```python
from build123d import *

# Parameters (mm, degrees)
SKETCH1_R           = 2.5
BOSS_EXTRUDE1_DEPTH = 2.54


with BuildPart() as part:
    # Sketch1 → Boss-Extrude1 (new body)
    with BuildSketch(Plane(origin=(0, 0, 0), x_dir=(1, 0, 0), z_dir=(0, 1, 0))):
        with BuildLine():
            Line((-127, 38.1), (-127, 23.495))
            ThreePointArc((-127, 23.495), (-124.768153673, 18.106846327), (-119.38, 15.875))
            Line((-119.38, 15.875), (119.38, 15.875))
            ThreePointArc((119.38, 15.875), (124.768153673, 18.106846327), (127, 23.495))
            Line((127, 23.495), (127, 38.1))
            Line((127, 38.1), (146.05, 38.1))
            Line((146.05, 38.1), (146.05, -38.1))
            Line((146.05, -38.1), (127, -38.1))
            Line((127, -38.1), (127, -15.875))
            Line((127, -15.875), (-127, -15.875))
            Line((-127, -15.875), (-127, -38.1))
            Line((-127, -38.1), (-146.05, -38.1))
            Line((-146.05, -38.1), (-146.05, 38.1))
            Line((-146.05, 38.1), (-127, 38.1))
        make_face()
        with Locations(Location((136.525, 20.32, 0), (0, 0, 270))):
            Circle(SKETCH1_R, mode=Mode.SUBTRACT)
        with Locations(Location((136.525, -20.32, 0), (0, 0, 270))):
            Circle(SKETCH1_R, mode=Mode.SUBTRACT)
        with Locations(Location((-136.525, 20.32, 0), (0, 0, 90))):
            Circle(SKETCH1_R, mode=Mode.SUBTRACT)
        with Locations(Location((-136.525, -20.32, 0), (0, 0, 90))):
            Circle(SKETCH1_R, mode=Mode.SUBTRACT)
    extrude(amount=BOSS_EXTRUDE1_DEPTH)


solid = part.part
```
Check sheet for the modelled part. Datum: model origin and axes. Units: mm. A direction names the side the tool comes from. Give positions to 0.01 mm unless a question says otherwise; leave off trailing zeros. Order: outer loops, then holes, each group sorted by start corner. A loop starts at its lowest first (then second) coordinate and runs counter-clockwise, first axis right, second up. Notation, with made-up numbers: M 62,2.5 L 92,2.5 A37 ccw 92,39.5 Z; hole C 72,31 d2. An arc over 180 degrees is marked long. Answer in a Markdown table with one row per item. Add a question column.
Q1. Sectioned sample at D-D, the plane x = 10. Record the boundary of the cut face in (y, z) (3 decimals).
Q2. Access from +Z, -Z, +X, -X, +Y, -Y to the whole of each face (thin tool, end or side, straight path). Record for faces 1 (the cylindrical face through (-124.83, 1.25, -18.17)), 2 (the flat face through (2, 0, -1)).
Q3. Sectioned sample at A-A, the plane z = 20.32. Record the boundary of the cut face in (x, y) (3 decimals).
Q4. Release check for a two-part mould opening along Z. For faces 3 (the flat face through (2, 2.54, -1)), 4 (the cylindrical face through (-139.004, 1.252, -19.995)), 5 (the cylindrical face through (124.71, 1.25, -18.05)) record: released by +Z, released by -Z, zero draft, split by the parting line, or undercut.
Q5. Sectioned sample at B-B, the plane y = 1.5. Record the boundary of the cut face in (x, z) (3 decimals), and give its area (3 significant figures).
Q6. Sectioned sample at C-C, the plane z = -20.32. Record the boundary of the cut face in (x, y) (3 decimals).
Q7. Gauge pin test, flat end, axial feed: pin 1 Ø4 at (x, z) = (136.525, -20.32) entering from +Y. Record the tip position at first contact, or that the pin passes through.
Q8. Thickness scan on L1, parallel to X at y = 1.3, z = 20.32 (3 decimals); L2, parallel to X at y = 1.65, z = -20.32 (3 decimals); L3, parallel to X at y = 0.6, z = 34.5. Record the ranges inside material, lowest first.
Verdict:
| question | item | result |
|---|---|---|
| 1 | outline | M 0,-15.875 L 2.54,-15.875 L 2.54,15.875 L 0,15.875 Z |
| 2 | face 1 | -Z, +Y, -Y |
| 2 | face 2 | +Z, -Z, +X, -X, -Y |
| 3 | outline | M -146.05,0 L -139.025,0 L -139.025,2.54 L -146.05,2.54 Z; M -134.025,0 L -127,0 L -127,2.54 L -134.025,2.54 Z; M 127,0 L 134.025,0 L 134.025,2.54 L 127,2.54 Z; M 139.025,0 L 146.05,0 L 146.05,2.54 L 139.025,2.54 Z |
| 4 | face 3 | zero draft |
| 4 | face 4 | undercut |
| 4 | face 5 | released by -Z |
| 5 | outline | M -146.05,-38.1 L -127,-38.1 L -127,-23.495 A7.62 cw -119.38,-15.875 L 119.38,-15.875 A7.62 cw 127,-23.495 L 127,-38.1 L 146.05,-38.1 L 146.05,38.1 L 127,38.1 L 127,15.875 L -127,15.875 L -127,38.1 L -146.05,38.1 Z; hole C -136.525,-20.32 d5; hole C -136.525,20.32 d5; hole C 136.525,-20.32 d5; hole C 136.525,20.32 d5 |
| 5 | area | 10,900 mm² |
| 6 | outline | M -146.05,0 L -139.025,0 L -139.025,2.54 L -146.05,2.54 Z; M -134.025,0 L -126.307,0 L -126.307,2.54 L -134.025,2.54 Z; M 126.307,0 L 134.025,0 L 134.025,2.54 L 126.307,2.54 Z; M 139.025,0 L 146.05,0 L 146.05,2.54 L 139.025,2.54 Z |
| 7 | pin 1 | through |
| 8 | L1 | -146.05 to -139.025, -134.025 to -127, 127 to 134.025, 139.025 to 146.05 |
| 8 | L2 | -146.05 to -139.025, -134.025 to -126.307, 126.307 to 134.025, 139.025 to 146.05 |
| 8 | L3 | -146.05 to -127, 127 to 146.05 |
